```python
from build123d import *

# Parameters (mm, degrees)
F1_DEPTH = 76.2


with BuildPart() as f1:
    # F0 (on Top) → F1 (new body)
    with BuildSketch(Plane.XY):
        with BuildLine():
            ThreePointArc((-0.635, 2.4593444248), (-1.5554259867, -2.0080463142), (2.54, 0))
            ThreePointArc((2.54, 0), (2.0080463142, 1.5554259867), (0.635, 2.4593444248))
            Line((0.635, 2.4593444248), (-0.635, 2.4593444248))
        make_face()
        with BuildLine():
            Line((-0.635, 2.4593444248), (0.635, 2.4593444248))
            ThreePointArc((0.635, 2.4593444248), (0, 2.54), (-0.635, 2.4593444248))
        make_face()
        with BuildLine():
            ThreePointArc((-0.635, 2.4593444248), (0, 2.54), (0.635, 2.4593444248))
            Line((0.635, 2.4593444248), (0.635, 3.7293444248))
            Line((0.635, 3.7293444248), (-0.635, 3.7293444248))
            Line((-0.635, 3.7293444248), (-0.635, 2.4593444248))
        make_face()
    extrude(amount=F1_DEPTH)


solid = f1.part
```
The listing builds one solid part. Answer for the finished solid, in the listing's coordinates (mm). Give positions to 0.01 mm unless a question says otherwise; leave off trailing zeros. Loops run counter-clockwise (first coordinate to the right, second up) from the corner with the lowest first, then second, coordinate; pieces in that order, holes last. Notation, with made-up numbers: (87.5, 24) - (105.5, 24) arc R20 cw to (105.5, 40) - close; hole circle Ø1 at (0, 16). An arc over 180 degrees is marked (long way). Return JSON: item names as keys, results as strings. Group by question number.
1. Straight lines are drawn through the part: line 1 (Y direction, x = -0.15, z = 40); line 2 (X direction, y = 3.25, z = 32) (3 decimals); line 3 (X direction, y = -0.25, z = 36.5). For each, find the intervals that lie inside material, in ascending order. Write a range as [from, to].
2. Determine the mould class of faces 1 (the flat face through (0, 3.729, 38)), 2 (the flat face through (-0.635, 3, 38)), 3 (the flat face through (0.635, 3, 38)) for opening direction X: pulls with the +X half, pulls with the -X half, needs draft (parallel to the pull), parting line crosses it, or undercut.
3. Find section A-A (z = 37). Write down the section's boundary in (x, y) (3 decimals), then the cut area to 3 significant figures.
4. Find section B-B (y = 1.5). Write down the section's boundary in (x, z).
5. Given pin 1 Ø0.6 at (y, z) = (3, 41.5) entering from +X (3 decimals); pin 2 Ø1.5 at (y, z) = (-1.5, 49) entering from -X; pin 3 Ø1.4 at (y, z) = (3, 27.5) entering from -X, each flat-ended and moving along its own axis, determine where each tip first touches the part or whether it passes through.
Verdict:
{
 "1": {"line 1": "y = [-2.54, 3.73]", "line 2": "x = [-0.635, 0.635]", "line 3": "x = [-2.53, 2.53]"},
 "2": {"face 1": "needs draft", "face 2": "pulls with the -X half", "face 3": "pulls with the +X half"},
 "3": {"outline": "(-0.635, 2.459) arc R2.54 ccw (long way) to (0.635, 2.459) - (0.635, 3.729) - (-0.635, 3.729) - close", "area": "21.8 mm^2"},
 "4": {"outline": "(-2.05, 0) - (2.05, 0) - (2.05, 76.2) - (-2.05, 76.2) - close"},
 "5": {"pin 1": "stops at x = 0.635", "pin 2": "stops at x = -2.43", "pin 3": "stops at x = -1.08"}
}
